```python
from build123d import *

# Parameters (mm, degrees)
F0_W      = 914.4
F0_H      = 38.1
F1_DEPTH  = 88.9
F2_W      = 88.9
F2_H      = 44.45
F2_W_2    = 469.9
F3_DEPTH  = 38.1
F4_W      = 88.9
F4_H      = 44.45
F4_H_2    = 869.95
F5_DEPTH  = 38.1
F6_R      = 6.35
F7_DEPTH  = 558.801
F9_W      = 25.4
F9_H      = 25.4
F10_DEPTH = 203.2
F11_W     = 25.4
F11_H     = 25.4
F12_DEPTH = 203.2
F13_R     = 6.35
F14_DEPTH = 406.4
F15_W     = 88.9
F15_H     = 38.1
F16_DEPTH = 381
F17_R     = 6.35
F18_DEPTH = 38.1
F19_W     = 25.4
F19_H     = 88.9
F20_DEPTH = 50.8
F21_R     = 12.7
F23_DEPTH = 25.4
F24_R     = 6.35
F25_DEPTH = 101.6
F26_W     = 88.9
F26_H     = 88.9
F27_DEPTH = 101.6
F28_W     = 469.9
F28_H     = 88.9
F28_W_2   = 558.8
F29_DEPTH = 25.4


with BuildPart() as f1:
    # F0 (on Right) → F1 (new body)
    with BuildSketch(Plane.YZ):
        with Locations((457.2, 19.05)):
            Rectangle(F0_W, F0_H)
    extrude(amount=F1_DEPTH)

    # F2 (on face) → F3 (join)
    with BuildSketch(Plane.XY.offset(38.1)):
        with Locations((44.45, 22.225)):
            Rectangle(F2_W, F2_H)
        with Locations((-234.95, 22.225)):
            Rectangle(F2_W_2, F2_H)
    extrude(amount=F3_DEPTH)

    # F4 (on face) → F5 (join)
    with BuildSketch(Plane(origin=(0, 0, 38.1), x_dir=(1, 0, 0), z_dir=(0, 0, -1))):
        with Locations((-425.45, -22.225)):
            Rectangle(F4_W, F4_H)
        with Locations((-425.45, -479.425)):
            Rectangle(F4_W, F4_H_2)
    extrude(amount=F5_DEPTH)

    # F6 (on face) → F7 (cut, through all)
    with BuildSketch(Plane(origin=(-469.9, 0, 0), x_dir=(0, -1, 0), z_dir=(-1, 0, 0))):
        with Locations((-133.35, 19.05)):
            Circle(F6_R)
    extrude(amount=-F7_DEPTH, mode=Mode.SUBTRACT)

    # F9 (on face) → F10 (join)
    with BuildSketch(Plane.XY.offset(38.1)):
        with Locations((12.7, 584.2)):
            Rectangle(F9_W, F9_H)
    extrude(amount=F10_DEPTH)

    # F11 (on face) → F12 (join)
    with BuildSketch(Plane.XY.offset(38.1)):
        with Locations((-393.7, 584.2)):
            Rectangle(F11_W, F11_H)
    extrude(amount=F12_DEPTH)

    # F13 (on face) → F14 (join)
    with BuildSketch(Plane(origin=(0, 0, 0), x_dir=(0, -1, 0), z_dir=(-1, 0, 0))):
        with Locations((-584.2, 228.6)):
            Circle(F13_R)
    extrude(amount=F14_DEPTH)

    # F15 (on face) → F16 (join)
    with BuildSketch(Plane(origin=(0, 0, 0), x_dir=(0, -1, 0), z_dir=(-1, 0, 0))):
        with Locations((-869.95, 19.05)):
            Rectangle(F15_W, F15_H)
    extrude(amount=F16_DEPTH)

    # F17 (on face) → F18 (cut)
    with BuildSketch(Plane.XY.offset(38.1)):
        with Locations((38.1, 863.6)):
            Circle(F17_R)
        with Locations((-419.1, 863.6)):
            Circle(F17_R)
    extrude(amount=-F18_DEPTH, mode=Mode.SUBTRACT)

    # F19 (on face) → F20 (join)
    with BuildSketch(Plane.XY.offset(38.1)):
        with Locations((-190.5, 869.95)):
            Rectangle(F19_W, F19_H)
    extrude(amount=F20_DEPTH)

    # F21
    f21_edges = [f1.edges().sort_by_distance(p)[0] for p in [
        (-336.55, 914.4, 38.1),
        (-44.45, 914.4, 38.1),
        (-190.5, 0, 76.2),
    ]]
    fillet(f21_edges, radius=F21_R)

    # F22 (on face) → F23 (cut)
    with BuildSketch(Plane(origin=(-203.2, 0, 0), x_dir=(0, -1, 0), z_dir=(-1, 0, 0))):
        Polygon((-825.5, 88.9), (-882.1451067924, 88.9), (-825.5, 38.1), align=None)
    extrude(amount=-F23_DEPTH, mode=Mode.SUBTRACT)

    # F24 (on face) → F25 (cut)
    with BuildSketch(Plane(origin=(0, 349.0370188612, -389.197622203), x_dir=(1, 0, 0), z_dir=(0, -0.667652347, 0.7444731987))):
        with Locations((-190.5, 697.0376830206)):
            Circle(F24_R)
    extrude(amount=-F25_DEPTH, mode=Mode.SUBTRACT)

    # F26 (on face) → F27 (join)
    with BuildSketch(Plane.XY.offset(38.1)):
        with Locations((-425.45, 215.9)):
            Rectangle(F26_W, F26_H)
        with Locations((44.45, 215.9)):
            Rectangle(F26_W, F26_H)
    extrude(amount=F27_DEPTH)

    # F28 (on face) → F29 (join)
    with BuildSketch(Plane.XY.offset(139.7)):
        with Locations((-146.05, 215.9)):
            Rectangle(F28_W, F28_H)
        with Locations((-190.5, 215.9)):
            Rectangle(F28_W_2, F28_H)
    extrude(amount=F29_DEPTH)


solid = f1.part
```
Can you work these out from the model? Positions are in its coordinate system, mm. A direction names the side the tool comes from. Round coordinates to 2 decimals unless told otherwise and drop trailing zeros. Order: outer loops, then holes, each group sorted by start corner. A loop starts at its lowest first (then second) coordinate and runs counter-clockwise, first axis right, second up.
(1) If we section it at B-B (y = 649.5): Please give me the cut outline in (x, z), plus the area to 3 significant figures.
Results are:
outline: (-469.9, 0) - (-381, 0) - (-381, 38.1) - (-469.9, 38.1) - close; (0, 0) - (88.9, 0) - (88.9, 38.1) - (0, 38.1) - close
area: 6,770 mm2
(2) We'd pull the mould along X, two halves only. Please class faces 6 (the face through (-193, 23, 38.1)), 7 (the face through (-187, 914.4, 14)), 8 (the face through (-406.4, 584, 138)), 9 (the face through (-193, 217, 139.7)): +X half, -X half, draft (parallel to the pull), parting line (faces both ways), or undercut.
Results are:
face 6: undercut
face 7: draft
face 8: -X half
face 9: undercut
(3) I'm going to push flat-ended pins straight in: pin 1 (12.5 mm diameter, centred on x = 14, z = 170, fed in from +Y); pin 2 (12.5 mm diameter, centred on x = -196, y = 891.5, fed in from +Z); pin 3 (2 mm diameter, centred on x = 20, z = 118, fed in from -Y). Where does each tip first touch, or does it pass through?
Results are:
pin 1: stops at y = 596.9
pin 2: stops at z = 88.9
pin 3: stops at y = 171.45
(4) On a 3-axis mill with a long thin cutter (end or side, diameter ignored), from which of +Z, -Z, +X, -X, +Y, -Y can I reach the whole of each face in a straight line? I mean faces 1 (the face through (-469.9, 387, 27)), 2 (the face through (-188, 825.5, 19)), 3 (the face through (-177.8, 879, 57)), 4 (the face through (13, 596.9, 138)), 5 (the face through (-394, 571.5, 138)). Say none if no direction works.
Results are:
face 1: +Z, -Z, -X, +Y, -Y
face 2: +Z, -Z, -Y
face 3: +Z, +X, +Y
face 4: +Z, +X, -X, +Y
face 5: +Z, +X, -X
(5) If we section it at A-A (x = -229.5): Please give me the cut outline in (y, z).
Results are:
outline: (0, 38.1) - (44.45, 38.1) - (44.45, 76.2) - (12.7, 76.2) arc R12.7 ccw to (0, 63.5) - close; (171.45, 139.7) - (260.35, 139.7) - (260.35, 165.1) - (171.45, 165.1) - close; circle Ø12.7 at (584.2, 228.6); (825.5, 0) - (914.4, 0) - (914.4, 25.4) arc R12.7 ccw to (901.7, 38.1) - (825.5, 38.1) - close
(6) If we section it at C-C (z = 174): Please give me the cut outline in (x, y), plus the area to 3 significant figures.
Results are:
outline: (-406.4, 571.5) - (-381, 571.5) - (-381, 596.9) - (-406.4, 596.9) - close; (0, 571.5) - (25.4, 571.5) - (25.4, 596.9) - (0, 596.9) - close
area: 1,290 mm2
(7) If I drill on L1, parallel to Y at x = 57, z = 19; L2, parallel to X at y = 863, z = 22; L3, parallel to X at y = 704.5, z = 20, over which ranges is the centre line in solid material (lowest first)?
Results are:
L1: y = 0 to 127, 139.7 to 914.4
L2: x = -469.9 to -425.42, -412.78 to 31.78, 44.42 to 88.9
L3: x = -469.9 to -381, 0 to 88.9
